from build123d import *

# Parameters (mm, degrees)
SZKIC1_W                                   = 50
SZKIC1_H                                   = 50
DODANIE_WYCI_GNI_CIE1_DEPTH                = 10
SZKIC2_W                                   = 5
SZKIC2_H                                   = 50
DODANIE_WYCI_GNI_CIE2_DEPTH                = 40
WYCI_CIE_WYCI_GNI_CIE_CIENKA_CIANKA2_DEPTH = 40


with BuildPart() as part:
    # Szkic1 → Dodanie-wyciągnięcie1 (new body)
    with BuildSketch(Plane.XY):
        Rectangle(SZKIC1_W, SZKIC1_H)
    extrude(amount=DODANIE_WYCI_GNI_CIE1_DEPTH)

    # Szkic2 → Dodanie-wyciągnięcie2 (add)
    with BuildSketch(Plane(origin=(0, 0, 0), x_dir=(-1, 0, 0), z_dir=(0, 0, -1))):
        with Locations((-6.5, 0)):
            Rectangle(SZKIC2_W, SZKIC2_H)
        with Locations((6.5, 0)):
            Rectangle(SZKIC2_W, SZKIC2_H)
    extrude(amount=DODANIE_WYCI_GNI_CIE2_DEPTH)

    # Szkic4 → Wycięcie-wyciągnięcie-cienka ścianka2 (cut)
    with BuildSketch(Plane(origin=(9, 0, 0), x_dir=(0, 0, -1), z_dir=(1, 0, 0))):
        with BuildLine():
            ThreePointArc((40, -5), (34.142135624, -19.142135624), (20, -25))
            Line((20, -25), (20, -35))
            ThreePointArc((20, -35), (41.213203436, -26.213203436), (50, -5))
            Line((50, -5), (40, -5))
        make_face()
        with BuildLine():
            ThreePointArc((20, 25), (34.142135624, 19.142135624), (40, 5))
            Line((40, 5), (50, 5))
            ThreePointArc((50, 5), (41.213203436, 26.213203436), (20, 35))
            Line((20, 35), (20, 25))
        make_face()
    extrude(amount=-WYCI_CIE_WYCI_GNI_CIE_CIENKA_CIANKA2_DEPTH, mode=Mode.SUBTRACT)


solid = part.part
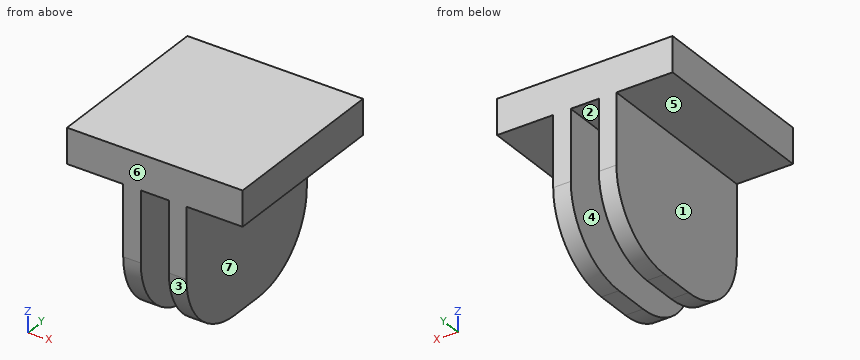
Check sheet for the modelled part. Datum: model origin and axes. Units: mm. Face numbers are marked on the shaded views. A direction names the side the tool comes from. Give positions to 0.01 mm unless a question says otherwise; leave off trailing zeros. Loops run counter-clockwise (first coordinate to the right, second up) from the corner with the lowest first, then second, coordinate; pieces in that order, holes last. Notation, with made-up numbers: M 84,64.5 L 125,64.5 A23 ccw 125,102.5 Z; hole C -38,68 d8. An arc over 180 degrees is marked long. Answer as a JSON object with one key per item and string values. Group by question number.
Q1. Go/stop test with flat-tipped pins: P1, Ø2, axis at x = -5.5, y = -11, coming from the -Z side; P2, Ø17.5, axis at x = -19.5, y = -1.5, coming from the -Z side; P3, Ø12, axis at y = 10.5, z = -28.5, coming from the -X side; P4, Ø4, axis at x = -14, z = -0.5, coming from the -Y side. Record where each tip stops, or that it passes through.
Q2. Cross-section at B-B on x = 5. Record the cut outline in (y, z).
Q3. Material ranges on line 1 along X through (y, z) = (-5, -34.5); line 2 along Z through (x, y) = (-17.5, 22.5); line 3 along Z through (x, y) = (-7, -5.5), recorded low to high. Write a range as [from, to].
Q4. Access from +Z, -Z, +X, -X, +Y, -Y to the whole of each face (thin tool, end or side, straight path). Record for the marked faces 4, 5, 6 and 7.
Q5. Cross-section at A-A on z = -18.5. Record the cut outline in (x, y), then the cut area to 3 significant figures.
Q6. Cross-section at D-D on z = -32. Record the cut outline in (x, y).
Q7. Cross-section at C-C on y = -12. Record the cut outline in (x, z) (3 decimals), then the cut area to 3 significant figures.
Q8. Release check for a two-part mould opening along X. For the marked faces 1, 2 and 3 record: released by +X, released by -X, zero draft, split by the parting line, or undercut.
Evaluation:
{
 "1": {"P1": "stops at z = -39.36", "P2": "stops at z = 0", "P3": "stops at x = -9", "P4": "stops at y = -25"},
 "2": {"outline": "M -25,-20 A20 ccw -5,-40 L 5,-40 A20 ccw 25,-20 L 25,10 L -25,10 Z"},
 "3": {"line 1": "x = [-9, -4], [4, 9]", "line 2": "z = [0, 10]", "line 3": "z = [-39.99, 10]"},
 "4": {"face 4": "-Z, +Y, -Y", "face 5": "-Z, -X, +Y, -Y", "face 6": "+Z, -Z, +X, -X, -Y", "face 7": "-Z, +X, +Y, -Y"},
 "5": {"outline": "M -9,-25 L -4,-25 L -4,25 L -9,25 Z; M 4,-25 L 9,-25 L 9,25 L 4,25 Z", "area": "500 mm2"},
 "6": {"outline": "M -9,-21 L -4,-21 L -4,21 L -9,21 Z; M 4,-21 L 9,-21 L 9,21 L 4,21 Z"},
 "7": {"outline": "M -25,0 L -9,0 L -9,-38.735 L -4,-38.735 L -4,0 L 4,0 L 4,-38.735 L 9,-38.735 L 9,0 L 25,0 L 25,10 L -25,10 Z", "area": "887 mm2"},
 "8": {"face 1": "released by -X", "face 2": "undercut", "face 3": "zero draft"}
}
